Can you work these out from the model? Positions are in its coordinate system, mm. Face numbers are marked on the shaded views. Coordinates: 2 decimals unless noted, no trailing zeros. Loops run counter-clockwise (first coordinate to the right, second up) from the corner with the lowest first, then second, coordinate; pieces in that order, holes last. Notation, with made-up numbers: (24, -28) -> (75, -28) arc R3 ccw to (75, -24) -> close; hole circle Ø9 at (45, 41.5). An arc over 180 degrees is marked (long way). Put each result on its own line as item: value. Start each with the question number.
Item 1: We'd pull the mould along Z, two halves only. Please class the marked faces 1, 2 and 3: pulls with the +Z half, pulls with the -Z half, needs draft (parallel to the pull), parting line crosses it, or undercut.
Item 2: Please list where these lines run through material, in increasing order: L1, parallel to Z at x = 61, y = 20.5; L2, parallel to Y at x = 78, z = -11.5; L3, parallel to Y at x = 42, z = 38.5. Write a range as from..to.
Item 3: If we section it at B-B on x = 12.5: Please give me the cut outline in (y, z).
Item 4: If we section it at C-C on z = 19: Please give me the cut outline in (x, y), plus the area to 3 significant figures.
Item 5: Will these pins go through, and if not, where does the flat tip stop? P1, Ø1, axis at x = 35.5, z = -22, coming from the -Y side; P2, Ø4, axis at x = 73.5, z = 36.5, coming from the +Y side.
Item 6: If we section it at A-A on y = 8.5: Please give me the cut outline in (x, z).
```python
from build123d import *

# Parameters (mm, degrees)
SALIENTE_EXTRUIR1_DEPTH = 100
CROQUIS2_W              = 10.010901807
CROQUIS2_H              = 4.106706179
CROQUIS2_W_2            = 28.903824567
SALIENTE_EXTRUIR2_DEPTH = 100


with BuildPart() as part:
    # Croquis1 → Saliente-Extruir1 (new body)
    with BuildSketch(Plane(origin=(0, 0, 0), x_dir=(0, 0, -1), z_dir=(1, 0, 0))):
        Polygon((-30, 3.5), (-40, 13.5), (40, 13.5), (30, 3.5), (50, 3.5), (50, 18.770945102), (-50, 18.770945102), (-50, 3.5), align=None)
    extrude(amount=SALIENTE_EXTRUIR1_DEPTH)

    # Croquis2 → Saliente-Extruir2 (add)
    with BuildSketch(Plane(origin=(100, 0, 0), x_dir=(0, 0, -1), z_dir=(1, 0, 0))):
        with Locations((-44.994549097, 20.824298192)):
            Rectangle(CROQUIS2_W, CROQUIS2_H)
        with Locations((-17.982777217, 20.824298192)):
            Rectangle(CROQUIS2_W_2, CROQUIS2_H)
        with Locations((17.982777217, 20.824298192)):
            Rectangle(CROQUIS2_W_2, CROQUIS2_H)
        with Locations((44.994549097, 20.824298192)):
            Rectangle(CROQUIS2_W, CROQUIS2_H)
    extrude(amount=-SALIENTE_EXTRUIR2_DEPTH)


solid = part.part
```
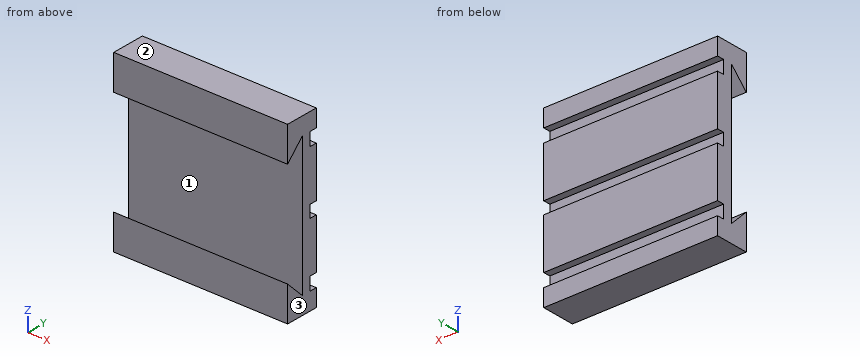
Solutions:
1. face 1: undercut
1. face 2: pulls with the +Z half
1. face 3: needs draft
2. L1: -50..-39.99, -32.43..-3.53, 3.53..32.43, 39.99..50
2. L2: 13.5..22.88
2. L3: 3.5..12, 13.5..18.77
3. outline: (3.5, -50) -> (22.88, -50) -> (22.88, -39.99) -> (18.77, -39.99) -> (18.77, -32.43) -> (22.88, -32.43) -> (22.88, -3.53) -> (18.77, -3.53) -> (18.77, 3.53) -> (22.88, 3.53) -> (22.88, 32.43) -> (18.77, 32.43) -> (18.77, 39.99) -> (22.88, 39.99) -> (22.88, 50) -> (3.5, 50) -> (3.5, 30) -> (13.5, 40) -> (13.5, -40) -> (3.5, -30) -> close
4. outline: (0, 13.5) -> (100, 13.5) -> (100, 22.88) -> (0, 22.88) -> close
4. area: 938 mm^2
5. P1: y = 13.5
5. P2: y = 18.77
6. outline: (0, -50) -> (100, -50) -> (100, -35) -> (0, -35) -> close; (0, 35) -> (100, 35) -> (100, 50) -> (0, 50) -> close
